Can you work these out from the model? Positions are in its coordinate system, mm. A direction names the side the tool comes from. Coordinates: 2 decimals unless noted, no trailing zeros. Loops run counter-clockwise (first coordinate to the right, second up) from the corner with the lowest first, then second, coordinate; pieces in that order, holes last. Notation, with made-up numbers: M 7.25,-12.75 L 60.25,-12.75 A18 ccw 60.25,19.25 Z; hole C 4.5,-26 d7. An arc over 180 degrees is marked long. Answer as a JSON object with one key per item and string values. Group by question number.
Item 1: Which directions (+Z, -Z, +X, -X, +Y, -Y) give clear straight access to the entire face, cutting with the end or side of a thin tool? Please do faces 4 (the flat face through (30, 25, -9)), 5 (the cylindrical face through (24.93, -25.78, 3.38)), 6 (the flat face through (10, -11, 11)).
Item 2: Suppose I cut it at A-A (z = 0). Write out the boundary of the cut face in (x, y), then the cut area to 3 significant figures.
Item 3: Suppose I cut it at D-D (z = 10.5). Write out the boundary of the cut face in (x, y), then the cut area to 3 significant figures.
Item 4: If I drill on line 1 (Y direction, x = 7.5, z = 0); line 2 (Y direction, x = 21.5, z = -9.5); line 3 (Z direction, x = 22, y = 4), over which ranges is the centre line in solid material (lowest first)?
Item 5: We'd pull the mould along X, two halves only. Please class faces 1 (the flat face through (0, -6.5, 0.2)), 2 (the flat face through (30, -6.5, 0.2)), 3 (the cylindrical face through (4.93, 0.66, -14.985)): +X half, -X half, draft (parallel to the pull), parting line (faces both ways), or undercut.
Item 6: I'm going to push flat-ended pins straight in: pin 1 Ø2 at (x, y) = (8.5, 13.5) entering from +Z; pin 2 Ø2 at (x, z) = (6, 3) entering from +Y; pin 3 Ø12 at (x, z) = (21, -13.5) entering from -Y; pin 4 Ø10 at (x, y) = (8, 2) entering from +Z. Where does each tip first touch, or does it pass through?
Item 7: Suppose I cut it at C-C (x = 3.75). Write out the boundary of the cut face in (y, z), then the cut area to 3 significant figures.
```python
from build123d import *

# Parameters (mm, degrees)
IZIM1_R                          = 15
Y_KSEKLIK_EKSTR_ZYON1_DEPTH      = 30
IZIM2_R                          = 10
KES_EKSTR_ZYON2_DEPTH            = 30
IZIM13_R                         = 30
Y_KSEKLIK_EKSTR_ZYON3_DEPTH      = 30
IZIM14_R                         = 26
KES_EKSTR_ZYON3_DEPTH            = 15
IZIM15_R                         = 15
Y_KSEKLIK_EKSTR_ZYON4_DEPTH      = 15
Y_KSEKLIK_EKSTR_ZYON4_DEPTH_BACK = 15
IZIM16_R                         = 10
KES_EKSTR_ZYON5_DEPTH            = 45
IZIM17_R                         = 26
KES_EKSTR_ZYON8_DEPTH            = 1
KES_EKSTR_ZYON8_DEPTH_BACK       = 15
IZIM19_R                         = 26
Y_KSEKLIK_EKSTR_ZYON5_DEPTH      = 5
Y_KSEKLIK_EKSTR_ZYON5_DEPTH_BACK = 5
IZIM20_R                         = 15
Y_KSEKLIK_EKSTR_ZYON6_DEPTH      = 10
IZIM21_R                         = 10
KES_EKSTR_ZYON9_DEPTH            = 55
IZIM24_R                         = 15
KES_EKSTR_ZYON10_DEPTH           = 15
IZIM26_R                         = 10
IZIM26_R_2                       = 6
Y_KSEKLIK_EKSTR_ZYON7_DEPTH      = 30


with BuildPart() as part:
    # Çizim1 → Yükseklik-Ekstrüzyon1 (new body)
    with BuildSketch(Plane(origin=(0, 0, 0), x_dir=(0, 0, -1), z_dir=(1, 0, 0))):
        Circle(IZIM1_R)
    extrude(amount=Y_KSEKLIK_EKSTR_ZYON1_DEPTH)

    # Çizim2 → Kes-Ekstrüzyon2 (cut)
    with BuildSketch(Plane.ZY):
        Circle(IZIM2_R)
    extrude(amount=-KES_EKSTR_ZYON2_DEPTH, mode=Mode.SUBTRACT)

    # Çizim13 → Yükseklik-Ekstrüzyon3 (add)
    with BuildSketch(Plane.ZY):
        Circle(IZIM13_R)
    extrude(amount=-Y_KSEKLIK_EKSTR_ZYON3_DEPTH)

    # Çizim14 → Kes-Ekstrüzyon3 (cut)
    with BuildSketch(Plane.ZY):
        Circle(IZIM14_R)
    extrude(amount=-KES_EKSTR_ZYON3_DEPTH, mode=Mode.SUBTRACT)

    # Çizim15 → Yükseklik-Ekstrüzyon4 (add, two sides)
    with BuildSketch(Plane.ZY) as y_kseklik_ekstr_zyon4_sk:
        Circle(IZIM15_R)
    extrude(amount=Y_KSEKLIK_EKSTR_ZYON4_DEPTH)
    extrude(y_kseklik_ekstr_zyon4_sk.sketch, amount=-Y_KSEKLIK_EKSTR_ZYON4_DEPTH_BACK)

    # Çizim16 → Kes-Ekstrüzyon5 (cut)
    with BuildSketch(Plane.ZY.offset(15)):
        Circle(IZIM16_R)
    extrude(amount=-KES_EKSTR_ZYON5_DEPTH, mode=Mode.SUBTRACT)

    # Çizim17 → Kes-Ekstrüzyon8 (cut, two sides)
    with BuildSketch(Plane(origin=(30, 0, 0), x_dir=(0, 0, -1), z_dir=(1, 0, 0))) as kes_ekstr_zyon8_sk:
        Circle(IZIM17_R)
    extrude(amount=KES_EKSTR_ZYON8_DEPTH, mode=Mode.SUBTRACT)
    extrude(kes_ekstr_zyon8_sk.sketch, amount=-KES_EKSTR_ZYON8_DEPTH_BACK, mode=Mode.SUBTRACT)

    # Çizim19 → Yükseklik-Ekstrüzyon5 (add, two sides)
    with BuildSketch(Plane.ZY.offset(-15)) as y_kseklik_ekstr_zyon5_sk:
        Circle(IZIM19_R)
    extrude(amount=Y_KSEKLIK_EKSTR_ZYON5_DEPTH)
    extrude(y_kseklik_ekstr_zyon5_sk.sketch, amount=-Y_KSEKLIK_EKSTR_ZYON5_DEPTH_BACK)

    # Çizim20 → Yükseklik-Ekstrüzyon6 (add)
    with BuildSketch(Plane(origin=(20, 0, 0), x_dir=(0, 0, -1), z_dir=(1, 0, 0))):
        Circle(IZIM20_R)
    extrude(amount=Y_KSEKLIK_EKSTR_ZYON6_DEPTH)

    # Çizim21 → Kes-Ekstrüzyon9 (cut)
    with BuildSketch(Plane.ZY.offset(15)):
        Circle(IZIM21_R)
    extrude(amount=-KES_EKSTR_ZYON9_DEPTH, mode=Mode.SUBTRACT)

    # Çizim24 → Kes-Ekstrüzyon10 (cut)
    with BuildSketch(Plane.ZY.offset(15)):
        Circle(IZIM24_R)
    extrude(amount=-KES_EKSTR_ZYON10_DEPTH, mode=Mode.SUBTRACT)

    # Çizim26 → Yükseklik-Ekstrüzyon7 (add)
    with BuildSketch(Plane(origin=(0, 0, 0), x_dir=(0, 0, -1), z_dir=(1, 0, 0))):
        Circle(IZIM26_R)
        Circle(IZIM26_R_2, mode=Mode.SUBTRACT)
    extrude(amount=Y_KSEKLIK_EKSTR_ZYON7_DEPTH)


solid = part.part
```
From the geometry:
{
 "1": {"face 4": "+Z, -Z, +X, +Y, -Y", "face 5": "+X", "face 6": "-X"},
 "2": {"outline": "M 0,-30 L 30,-30 L 30,-26 L 20,-26 L 20,-15 L 30,-15 L 30,-6 L 0,-6 L 0,-15 L 10,-15 L 10,-26 L 0,-26 Z; M 0,6 L 30,6 L 30,15 L 20,15 L 20,26 L 30,26 L 30,30 L 0,30 L 0,26 L 10,26 L 10,15 L 0,15 Z", "area": "1,000 mm2"},
 "3": {"outline": "M 0,-28.1 L 30,-28.1 L 30,-23.79 L 20,-23.79 L 20,-10.71 L 30,-10.71 L 30,10.71 L 20,10.71 L 20,23.79 L 30,23.79 L 30,28.1 L 0,28.1 L 0,23.79 L 10,23.79 L 10,10.71 L 0,10.71 L 0,-10.71 L 10,-10.71 L 10,-23.79 L 0,-23.79 Z", "area": "1,160 mm2"},
 "4": {"line 1": "-30 to -26, -15 to -6, 6 to 15, 26 to 30", "line 2": "-28.46 to -24.2, -11.61 to 11.61, 24.2 to 28.46", "line 3": "-29.73 to -25.69, -14.46 to -4.47, 4.47 to 14.46, 25.69 to 29.73"},
 "5": {"face 1": "-X half", "face 2": "+X half", "face 3": "draft"},
 "6": {"pin 1": "z = 27.27", "pin 2": "y = 29.93", "pin 3": "y = -29.05", "pin 4": "z = 30"},
 "7": {"outline": "C 0,0 d60; C 0,0 d30; hole C 0,0 d52; hole C 0,0 d12", "area": "1,300 mm2"}
}
